Drawing for the job (mm, zero at the part's lowest x, y, z). Round coordinates to 2 decimals unless told otherwise and drop trailing zeros. Loops run counter-clockwise (first coordinate to the right, second up) from the corner with the lowest first, then second, coordinate; pieces in that order, holes last. Notation, with made-up numbers: (78, 43) -> (124, 43) arc R31 cw to (124, 68) -> close; hole circle Ø11 at (74.25, 55). An arc over 180 degrees is marked (long way). Put each result on its own line as item: value. Start each with the question number.
Item 1: Drill centre lines: probe 1 along X at (y, z) = (65, 10.25); probe 2 along X at (y, z) = (67, 16.5); probe 3 along Z at (x, y) = (6, 81). Where is each one in solid material? Low to high. Write a range as [from, to].
Item 2: Flat gauge pins, fed straight in: pin 1 Ø6.5 at (y, z) = (4, 6) entering from -X (3 decimals); pin 2 Ø9 at (x, z) = (75, 12.5) entering from -Y; pin 3 Ø5 at (x, z) = (17, 8.5) entering from -Y; pin 4 Ø4 at (x, z) = (50.5, 10.5) entering from +Y. Where does each tip first touch, or does it go through?
Item 3: Cut at C-C, the plane y = 69.5. List the corners of the cut face in (x, z), plus the area to 3 significant figures.
Item 4: Cut at D-D, the plane x = 65.5. List the corners of the cut face in (y, z), plus the area to 3 significant figures.
Item 5: Cut at A-A, the plane z = 11.75. List the corners of the cut face in (x, y) (3 decimals), plus the area to 3 significant figures.
Item 6: Pull direction Z, two halves, no side cores. Call the marked faces 1, 2 and 3: +Z half, -Z half, draft (parallel to the pull), parting line (faces both ways), or undercut.
Item 7: Cut at B-B, the plane z = 2.25. List the corners of the cut face in (x, y) (3 decimals).
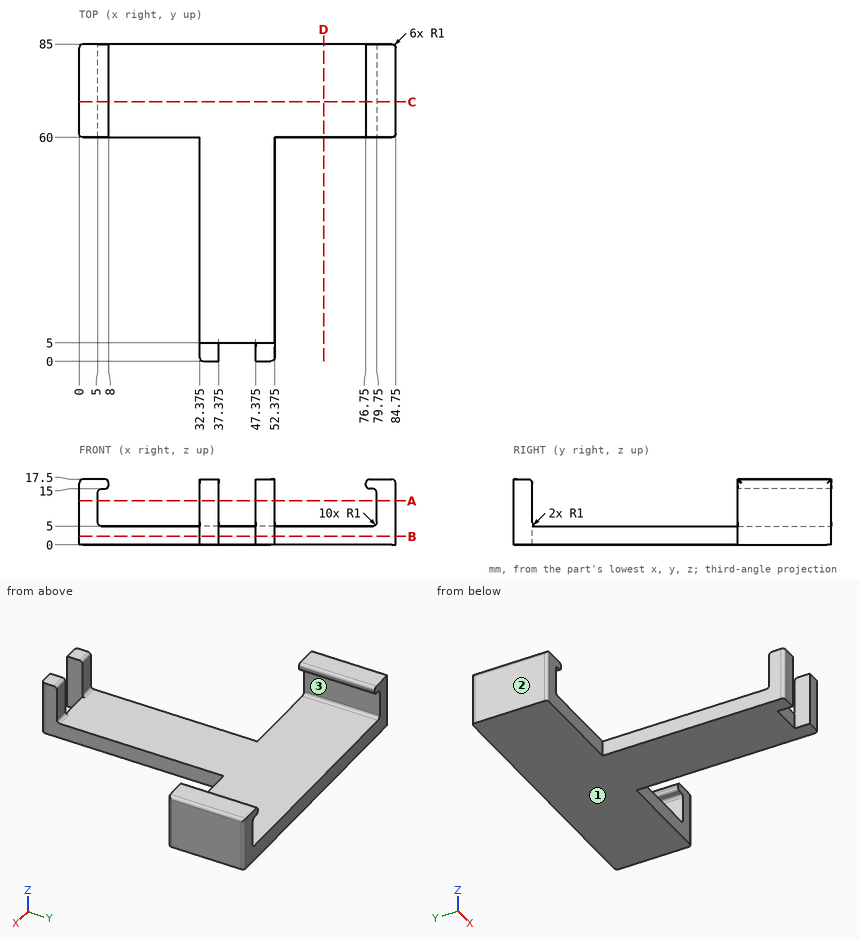
Reply:
1. probe 1: x = [0, 5], [79.75, 84.75]
1. probe 2: x = [0, 8], [76.75, 84.75]
1. probe 3: z = [0, 5], [15, 17.5]
2. pin 1: stops at x = 32.375
2. pin 2: stops at y = 60
2. pin 3: passes through
2. pin 4: stops at y = 5
3. outline: (0, 0) -> (84.75, 0) -> (84.75, 16.5) arc R1 ccw to (83.75, 17.5) -> (77.75, 17.5) arc R1 ccw to (76.75, 16.5) -> (76.75, 16) arc R1 ccw to (77.75, 15) -> (78.75, 15) arc R1 cw to (79.75, 14) -> (79.75, 6) arc R1 cw to (78.75, 5) -> (6, 5) arc R1 cw to (5, 6) -> (5, 14) arc R1 cw to (6, 15) -> (7, 15) arc R1 ccw to (8, 16) -> (8, 16.5) arc R1 ccw to (7, 17.5) -> (1, 17.5) arc R1 ccw to (0, 16.5) -> close
3. area: 563 mm^2
4. outline: (60, 0) -> (85, 0) -> (85, 5) -> (60, 5) -> close
4. area: 125 mm^2
5. outline: (0, 61) arc R1 ccw to (1, 60) -> (5, 60) -> (5, 85) -> (1, 85) arc R1 ccw to (0, 84) -> close; (32.375, 1) arc R1 ccw to (33.375, 0) -> (37.375, 0) -> (37.375, 5) -> (32.375, 5) -> close; (47.375, 0) -> (51.375, 0) arc R1 ccw to (52.375, 1) -> (52.375, 5) -> (47.375, 5) -> close; (79.75, 60) -> (83.75, 60) arc R1 ccw to (84.75, 61) -> (84.75, 84) arc R1 ccw to (83.75, 85) -> (79.75, 85) -> close
5. area: 299 mm^2
6. face 1: -Z half
6. face 2: draft
6. face 3: undercut
7. outline: (0, 61) arc R1 ccw to (1, 60) -> (32.375, 60) -> (32.375, 1) arc R1 ccw to (33.375, 0) -> (37.375, 0) -> (37.375, 5) -> (47.375, 5) -> (47.375, 0) -> (51.375, 0) arc R1 ccw to (52.375, 1) -> (52.375, 60) -> (83.75, 60) arc R1 ccw to (84.75, 61) -> (84.75, 84) arc R1 ccw to (83.75, 85) -> (1, 85) arc R1 ccw to (0, 84) -> close
